Build history of the part. All positions in model axes, mm. Coordinates: 2 decimals unless noted, no trailing zeros. Order: outer loops, then holes, each group sorted by start corner. A loop starts at its lowest first (then second) coordinate and runs counter-clockwise, first axis right, second up. Notation, with made-up numbers: (-4, 85) - (48, 85) arc R26 cw to (48, 118) - close; hole circle Ø5 at (9, 57). An arc over 180 degrees is marked (long way). Return JSON: item names as keys, results as strings.
Autodesk Inventor part; units mm, degrees
ref_plane "YZ Plane" through (0, 0, 0) normal (1, 0, 0) x (0, 1, 0)
ref_plane "XZ Plane" through (0, 0, 0) normal (0, 1, 0) x (-1, 0, 0)
ref_plane "XY Plane" through (0, 0, 0) normal (0, 0, 1) x (1, 0, 0)
sketch "スケッチ1" plane through (0, 0, 0) normal (1, 0, 0) x (0, 1, 0)
  line L0 (-40, 200) -> (-90, 200)
  line L1 (-90, 200) -> (-90, -200)
  line L2 (-90, -200) -> (90, -200)
  line L3 (90, -200) -> (90, -78.7859)
  line L4 (90, -78.7859) -> (-40, 200)
  line L5 (-126, 0) -> (126, 0)
  line L6 (0, -280) -> (0, 280)
  point P0 (0, 0)
  point P1 (-90, 0)
  point P2 (0, -200)
  dimension "d0" = 400
  dimension "d1" = 50
  dimension "d2" = 180
  dimension "d3" = 25
extrude "押し出し1" add sketch "スケッチ1" along normal blind 3
properties part number "stay" material "アルミニウム 6061"
1. Cut at C-C on y = 71.5. Give the cut face in (x, z), plus the area to 3 significant figures.
Check values:
{"outline": "(0, -200) - (3, -200) - (3, -39.11) - (0, -39.11) - close", "area": "483 mm²"}
2. Probe L1, parallel to Y at x = 2.1, z = -60; L2, parallel to Z at x = 1.9, y = 40.5; L3, parallel to Y at x = 2.8, z = 60.5. List the from-to ranges inside material, lowest first.
Check values:
{"L1": "-90 to 81.24", "L2": "-200 to 27.37", "L3": "-90 to 25.05"}
3. Cut at B-B on z = -60. Give the cut face in (x, y).
Check values:
{"outline": "(0, -90) - (3, -90) - (3, 81.24) - (0, 81.24) - close"}
4. Cut at A-A on x = 2.5. Give the cut face in (y, z), plus the area to 3 significant figures.
Check values:
{"outline": "(-90, -200) - (90, -200) - (90, -78.79) - (-40, 200) - (-90, 200) - close", "area": "53,900 mm²"}
